Geometry check sheet. Reference: the model listing, model coordinates, mm. A direction names the side the tool comes from. Give positions to 0.01 mm unless a question says otherwise; leave off trailing zeros. Write each loop counter-clockwise with the first axis right and the second up, starting at its lowest first coordinate (ties: lowest second). Pieces come first, ordered by that corner, then holes. Notation, with made-up numbers: (86.5, -8) -> (135.5, -8) arc R4 ccw to (135.5, -3) -> close; hole circle Ø6 at (71, 83.5). An arc over 180 degrees is marked (long way). Write item = value, one per line. Start each with the question number.
1. Cross-section at A-A, the plane z = 9. Record the cut outline in (x, y).
2. Cross-section at C-C, the plane x = 10.5. Record the cut outline in (y, z).
3. Cross-section at D-D, the plane y = 8. Record the cut outline in (x, z).
4. Thickness scan on line 1 along Z through (x, y) = (-10.5, 22); line 2 along X through (y, z) = (13.5, 12.25); line 3 along X through (y, z) = (15, 10). Record the ranges inside material, lowest first.
5. Mould release check, pull along Y, two halves, no side actions. Record for faces 1 (the flat face through (0, 7, 0)), 2 (the flat face through (-14, 39, 9)), 3 (the cylindrical face through (-14.43, 22.903, 9.513)): pulls with the +Y half, pulls with the -Y half, needs draft (parallel to the pull), parting line crosses it, or undercut.
6. Cross-section at B-B, the plane y = 19. Record the cut outline in (x, z).
7. Set-up check for faces 4 (the cylindrical face through (-17.05, 8.11, 8.89)), 5 (the flat face through (0, 10, 9)), 6 (the flat face through (19.5, 19.2, 4.9)): record each of +Z, -Z, +X, -X, +Y, -Y from which the full face is reachable in a straight line by a thin tool's end or side.
```python
from build123d import *

# Parameters (mm, degrees)
BOSS_EXTRUDE1_DEPTH         = 18
SKETCH3_R                   = 3.937
CUT_EXTRUDE1_DEPTH          = 40
F_1_4_20_TAPPED_HOLE1_D     = 5.1054
F_1_4_20_TAPPED_HOLE1_DEPTH = 19.05
F_1_4_20_TAPPED_HOLE1_TIP   = 1.533816902


with BuildPart() as part:
    # Sketch1 → Boss-Extrude1 (new body)
    with BuildSketch(Plane.XY):
        Polygon((-19.5, 0), (19.5, 0), (19.5, 39), (9.5, 39), (9.5, 10), (-9.5, 10), (-9.5, 39), (-19.5, 39), align=None)
    extrude(amount=BOSS_EXTRUDE1_DEPTH)

    # Sketch3 → Cut-Extrude1 (cut, through all)
    with BuildSketch(Plane(origin=(19.5, 0, 0), x_dir=(0, 0, -1), z_dir=(1, 0, 0))):
        with Locations((-9, 19)):
            Circle(SKETCH3_R)
    extrude(amount=-CUT_EXTRUDE1_DEPTH, mode=Mode.SUBTRACT)

    # 1/4-20 Tapped Hole1
    with Locations(Plane(origin=(0, 0, 0), x_dir=(-1, 0, 0), z_dir=(0, -1, 0))):
        with Locations((-14.5, -9), (14.5, -9)):
            Hole(F_1_4_20_TAPPED_HOLE1_D / 2, depth=F_1_4_20_TAPPED_HOLE1_DEPTH)
            with Locations((0, 0, -(F_1_4_20_TAPPED_HOLE1_DEPTH + F_1_4_20_TAPPED_HOLE1_TIP / 2))):  # 118° drill point
                Cone(0, F_1_4_20_TAPPED_HOLE1_D / 2, F_1_4_20_TAPPED_HOLE1_TIP, mode=Mode.SUBTRACT)


solid = part.part
```
Answers:
q1.outline = (-19.5, 0) -> (-17.05, 0) -> (-17.05, 15.06) -> (-19.5, 15.06) -> close; (-19.5, 22.94) -> (-9.5, 22.94) -> (-9.5, 39) -> (-19.5, 39) -> close; (-11.95, 0) -> (11.95, 0) -> (11.95, 15.06) -> (9.5, 15.06) -> (9.5, 10) -> (-9.5, 10) -> (-9.5, 15.06) -> (-11.95, 15.06) -> close; (9.5, 22.94) -> (19.5, 22.94) -> (19.5, 39) -> (9.5, 39) -> close; (17.05, 0) -> (19.5, 0) -> (19.5, 15.06) -> (17.05, 15.06) -> close
q2.outline = (0, 0) -> (39, 0) -> (39, 18) -> (0, 18) -> close; hole circle Ø7.87 at (19, 9)
q3.outline = (-19.5, 0) -> (19.5, 0) -> (19.5, 18) -> (-19.5, 18) -> close; hole circle Ø5.11 at (-14.5, 9); hole circle Ø5.11 at (14.5, 9)
q4.line_1 = 0 to 6.45, 11.55 to 18
q4.line_2 = -19.5 to -9.5, 9.5 to 19.5
q4.line_3 = -19.5 to -16.85, -12.15 to -9.5, 9.5 to 12.15, 16.85 to 19.5
q5.face_1 = needs draft
q5.face_2 = pulls with the +Y half
q5.face_3 = undercut
q6.outline = (-19.5, 0) -> (-9.5, 0) -> (-9.5, 5.06) -> (-19.5, 5.06) -> close; (-19.5, 12.94) -> (-9.5, 12.94) -> (-9.5, 18) -> (-19.5, 18) -> close; (9.5, 0) -> (19.5, 0) -> (19.5, 5.06) -> (9.5, 5.06) -> close; (9.5, 12.94) -> (19.5, 12.94) -> (19.5, 18) -> (9.5, 18) -> close
q7.face_4 = -Y
q7.face_5 = +Z, -Z, +Y
q7.face_6 = +Z, -Z, +X, +Y, -Y
